from build123d import *

# Parameters (mm, degrees)
BOSS_EXTRUDE1_DEPTH = 15
SKETCH11_R          = 1.75
CUT_EXTRUDE1_DEPTH  = 15
SKETCH12_R          = 3
CUT_EXTRUDE2_DEPTH  = 2
CHAMFER1_SIZE       = 2
CHAMFER1_SIZE2      = 5
CHAMFER2_SIZE       = 5
CHAMFER2_SIZE2      = 2
SKETCH13_W          = 3
SKETCH13_H          = 5
CUT_EXTRUDE3_DEPTH  = 36
FILLET1_R           = 7


with BuildPart() as part:
    # Sketch1 → Boss-Extrude1 (new body)
    with BuildSketch(Plane(origin=(0, 0, 0), x_dir=(1, 0, 0), z_dir=(0, 1, 0))):
        Polygon((-15, 0), (15, 0), (15, 5), (5, 5), (2.113248654, 10), (-2.113248654, 10), (-5, 5), (-15, 5), align=None)
    extrude(amount=BOSS_EXTRUDE1_DEPTH)

    # Sketch11 → Cut-Extrude1 (cut)
    with BuildSketch(Plane(origin=(0, 0, -5), x_dir=(-1, 0, 0), z_dir=(0, 0, -1))):
        with Locations((-10, 7.5)):
            Circle(SKETCH11_R)
        with Locations((10, 7.5)):
            Circle(SKETCH11_R)
    extrude(amount=-CUT_EXTRUDE1_DEPTH, mode=Mode.SUBTRACT)

    # Sketch12 → Cut-Extrude2 (cut)
    with BuildSketch(Plane(origin=(0, 0, -5), x_dir=(-1, 0, 0), z_dir=(0, 0, -1))):
        with Locations((-10, 7.5)):
            Circle(SKETCH12_R)
        with Locations((10, 7.5)):
            Circle(SKETCH12_R)
    extrude(amount=-CUT_EXTRUDE2_DEPTH, mode=Mode.SUBTRACT)

    # Chamfer1
    chamfer1_edges = [part.edges().sort_by_distance(p)[0] for p in [
        (0, 15, -10),
    ]]
    chamfer1_side = [part.faces().sort_by_distance(p)[0] for p in [
        (0, 7.5, -10),
    ]]
    chamfer(chamfer1_edges, length=CHAMFER1_SIZE, length2=CHAMFER1_SIZE2, reference=chamfer1_side[0])

    # Chamfer2
    chamfer2_edges = [part.edges().sort_by_distance(p)[0] for p in [
        (0, 0, -10),
    ]]
    chamfer2_side = [part.faces().sort_by_distance(p)[0] for p in [
        (0, 0, -3.3934981),
    ]]
    chamfer(chamfer2_edges, length=CHAMFER2_SIZE, length2=CHAMFER2_SIZE2, reference=chamfer2_side[0])

    # Sketch13 → Cut-Extrude3 (cut, through all)
    with BuildSketch(Plane(origin=(15, 0, 0), x_dir=(0, 0, -1), z_dir=(1, 0, 0))):
        with Locations((6.5, 7.5)):
            Rectangle(SKETCH13_W, SKETCH13_H)
    extrude(amount=-CUT_EXTRUDE3_DEPTH, mode=Mode.SUBTRACT)

    # Fillet1
    fillet1_edges = [part.edges().sort_by_distance(p)[0] for p in [
        (15, 15, -2.5),
        (-15, 0, -2.5),
        (-15, 15, -2.5),
        (15, 0, -2.5),
    ]]
    fillet(fillet1_edges, radius=FILLET1_R)


solid = part.part
Verification items for the finished model (mm, model axes). A direction names the side the tool comes from. Coordinates: 2 decimals unless noted, no trailing zeros. Loops run counter-clockwise (first coordinate to the right, second up) from the corner with the lowest first, then second, coordinate; pieces in that order, holes last. Notation, with made-up numbers: M 5,63 L 27,63 A16 cw 27,80 Z; hole C 21.5,-34.5 d6. An arc over 180 degrees is marked long. One line per item, written item: value.
1. Material ranges on line 1 along X through (y, z) = (7.5, -3.35); line 2 along Z through (x, y) = (0.75, 8.5); line 3 along X through (y, z) = (6.75, -0.5), recorded low to high. Write a range as from..to.
Answers follow:
line 1: -15..-13, -7..7, 13..15
line 2: -10..-8, -5..0
line 3: -15..-11.58, -8.42..8.42, 11.58..15
2. Mould release check, pull along Z, two halves, no side actions. Record for faces 1 (the flat face through (0, 5, -6)), 2 (the flat face through (-15, 7.5, -2.5)), 3 (the flat face through (0, 7, 0)): pulls with the +Z half, pulls with the -Z half, needs draft (parallel to the pull), parting line crosses it, or undercut.
Answers follow:
face 1: undercut
face 2: needs draft
face 3: pulls with the +Z half
3. Gauge pin test, flat ends, axial feed: P1, Ø5.5, axis at x = 10, y = 7.5, coming from the -Z side; P2, Ø5, axis at y = 11.5, z = -2, coming from the -X side; P3, Ø2.5, axis at x = 2, z = -6.5, coming from the -Y side. Record the tip position at first contact, or that the pin passes through.
Answers follow:
P1: z = -3
P2: x = -14.93
P3: y = 0.1
4. Set-up check for faces 4 (the flat face through (-12, 8, -3)), 5 (the flat face through (0, 10, -6)), 6 (the cylindrical face through (-12.9, 13, -2.5)): record each of +Z, -Z, +X, -X, +Y, -Y from which the full face is reachable in a straight line by a thin tool's end or side.
Answers follow:
face 4: -Z
face 5: +X, -X
face 6: +Z, -Z, -X, +Y
5. Section check C-C on x = -1.25. Record the cut outline in (y, z), plus the area to 3 significant figures.
Answers follow:
outline: M 0,-5 L 2,-10 L 13,-10 L 15,-5 L 15,0 L 0,0 Z; hole M 5,-8 L 10,-8 L 10,-5 L 5,-5 Z
area: 125 mm^2
6. Section check B-B on z = -3.75. Record the cut outline in (x, y), plus the area to 3 significant figures.
Answers follow:
outline: M -15,7 A7 ccw -8,0 L 8,0 A7 ccw 15,7 L 15,8 A7 ccw 8,15 L -8,15 A7 ccw -15,8 Z; hole C -10,7.5 d6; hole C 10,7.5 d6
area: 351 mm^2
7. Section check A-A on y = 7.5. Record the cut outline in (x, z).
Answers follow:
outline: M -15,-5 L -13,-5 L -13,-3 L -11.75,-3 L -11.75,0 L -15,0 Z; M -8.25,-3 L -7,-3 L -7,-5 L 7,-5 L 7,-3 L 8.25,-3 L 8.25,0 L -8.25,0 Z; M -3.27,-8 L -2.11,-10 L 2.11,-10 L 3.27,-8 Z; M 11.75,-3 L 13,-3 L 13,-5 L 15,-5 L 15,0 L 11.75,0 Z
8. Section check D-D on x = 9.75. Record the cut outline in (y, z), plus the area to 3 significant figures.
Answers follow:
outline: M 0.22,-5 L 4.51,-5 L 4.51,-3 L 5.77,-3 L 5.77,0 L 0.22,0 Z; M 9.23,-3 L 10.49,-3 L 10.49,-5 L 14.78,-5 L 14.78,0 L 9.23,0 Z
area: 50.4 mm^2
